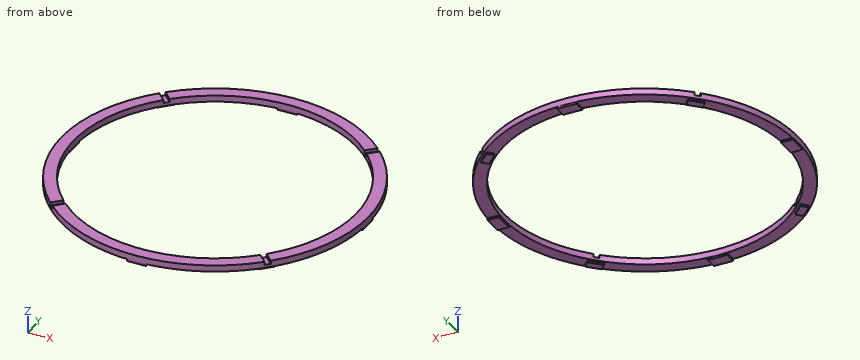
from build123d import *

# Parameters (mm, degrees)
F0_R            = 78.74
F0_R_2          = 72.39
F1_DEPTH        = 3.25
F3_DEPTH        = 1.63
F3_COPIES_COUNT = 4
F6_DEPTH        = 1
F7_COUNT        = 4
F7_ANGLE        = 270
F9_DEPTH        = 1
F10_COUNT       = 4
F10_ANGLE       = 270


# Not quite as in the source:
# - a feature of the source that left no trace in its solid (it failed there, or was rolled back) is left out
# - a pattern or mirror of a feature is missing from the dataset's text; its kind, count and spacing are read off the source's solid


with BuildPart() as f1:
    # F0 (on Top) → F1 (new body)
    with BuildSketch(Plane.XY):
        Circle(F0_R)
        Circle(F0_R_2, mode=Mode.SUBTRACT)
    extrude(amount=F1_DEPTH)

    # F2 (on face) → F3 (cut)
    with BuildSketch(Plane.XY.offset(3.25)):
        with BuildLine():
            Line((-50.1158095189, 52.2371298624), (-54.6068240538, 56.7281443973))
            ThreePointArc((-54.6068240538, 56.7281443973), (-55.6775879506, 55.6775879506), (-56.7281443973, 54.6068240538))
            Line((-56.7281443973, 54.6068240538), (-52.2371298624, 50.1158095189))
            ThreePointArc((-52.2371298624, 50.1158095189), (-51.1874598901, 51.1874598901), (-50.1158095189, 52.2371298624))
        make_face()
    f3 = extrude(amount=-F3_DEPTH, mode=Mode.SUBTRACT)

    # F3_copies: F3 ×4 about axis
    f3_copies_axis = Axis((0, 0, 0), (0, 0, 1))
    for i in range(1, F3_COPIES_COUNT):
        add(f3.rotate(f3_copies_axis, i * 360 / F3_COPIES_COUNT), mode=Mode.SUBTRACT)

    # F5 (on face) → F6 (join)
    with BuildSketch(Plane(origin=(0, 0, 0), x_dir=(1, 0, 0), z_dir=(0, 0, -1))):
        Polygon((-54.8467374827, 49.1898832332), (-52.018310358, 52.018310358), (-54.8467374827, 54.8467374827), (-57.6751646075, 52.018310358), (-56.2609510451, 50.6040967956), align=None)
        Polygon((-54.8467374827, 54.8467374827), (-52.018310358, 52.018310358), (-49.1898832332, 54.8467374827), (-50.6040967956, 56.2609510451), (-52.018310358, 57.6751646075), align=None)
    f6 = extrude(amount=F6_DEPTH)

    # F7: F6 ×4 about axis
    f7_axis = Axis((0, 0, 0), (0, 0, -1))
    for i in range(1, F7_COUNT):
        add(f6.rotate(f7_axis, i * F7_ANGLE / (F7_COUNT - 1)))

    # F8 (on face) → F9 (join)
    with BuildSketch(Plane(origin=(0, 0, 0), x_dir=(1, 0, 0), z_dir=(0, 0, -1))):
        Polygon((-5, 78.565), (-5, 75.565), (-5, 72.565), (0, 72.565), (5, 72.565), (5, 75.565), (5, 78.565), (0, 78.565), align=None)
    f9 = extrude(amount=F9_DEPTH)

    # F10: F9 ×4 about axis
    f10_axis = Axis((0, 0, 0), (0, 0, 1))
    for i in range(1, F10_COUNT):
        add(f9.rotate(f10_axis, i * F10_ANGLE / (F10_COUNT - 1)))


solid = f1.part
Geometry: final body of the model. Coordinates: model frame, mm. Round coordinates to 2 decimals unless told otherwise and drop trailing zeros. Loops run counter-clockwise (first coordinate to the right, second up) from the corner with the lowest first, then second, coordinate; pieces in that order, holes last. Notation, with made-up numbers: M 51.5,-23 L 102.5,-23 A7 ccw 102.5,-14 Z; hole C 72,-21 d2. An arc over 180 degrees is marked long. Put each result on its own line as item: value. Start each with the question number.
(1) Section query A-A (y = 0). Return loops of the section in (x, z) (3 decimals).
(2) Material intervals for line 1 along X through (y, z) = (2, 1.6); line 2 along Y through (x, z) = (0, 1.8); line 3 along Y through (x, z) = (35, 2.9), sorted ascending. Write a range as [from, to].
(3) Contact query for flat-ended pins moving along their axis: pin 1 Ø1.1 at (y, z) = (-2.5, -0.5) entering from -X; pin 2 Ø0.8 at (x, z) = (74, -0.5) entering from -Y; pin 3 Ø0.5 at (x, z) = (1.5, -0.5) entering from -Y (3 decimals). Output: stop coordinate, or through.
(4) Section query C-C (y = 37). Return loops of the section in (x, z), then the cut area to 3 significant figures.
(5) Section query D-D (x = 68.5). Return loops of the section in (y, z), then the cut area to 3 significant figures.
Findings below:
1. outline: M -78.74,0 L -78.565,0 L -78.565,-1 L -72.565,-1 L -72.565,0 L -72.39,0 L -72.39,3.25 L -78.74,3.25 Z; M 72.39,0 L 72.565,0 L 72.565,-1 L 78.565,-1 L 78.565,0 L 78.74,0 L 78.74,3.25 L 72.39,3.25 Z
2. line 1: x = [-78.71, -72.36], [72.36, 78.71]
2. line 2: y = [-78.74, -72.39], [72.39, 78.74]
2. line 3: y = [-70.53, -63.37], [63.37, 70.53]
3. pin 1: stops at x = -78.71
3. pin 2: stops at y = -5
3. pin 3: stops at y = -78.565
4. outline: M -69.51,0 L -62.22,0 L -62.22,3.25 L -69.51,3.25 Z; M 62.22,0 L 69.51,0 L 69.51,3.25 L 62.22,3.25 Z
4. area: 47.4 mm2
5. outline: M -38.83,0 L -23.41,0 L -23.41,3.25 L -38.83,3.25 Z; M 23.41,0 L 38.83,0 L 38.83,3.25 L 23.41,3.25 Z
5. area: 100 mm2
